For this review, take the finished solid that the model builds, in its own axes (mm). A direction names the side the tool comes from. Coordinates: 2 decimals unless noted, no trailing zeros. Order: outer loops, then holes, each group sorted by start corner. A loop starts at its lowest first (then second) coordinate and runs counter-clockwise, first axis right, second up. Notation, with made-up numbers: (45.5, 85) -> (81.5, 85) arc R20 ccw to (81.5, 112) -> close; hole circle Ø10 at (-16.5, 62). An arc over 180 degrees is marked (long way). Return JSON: item names as keys, results as strings. Group by question number.
Item 1: Take a section at C-C (x = 1262). Write out the cut boundary in (y, z), then the cut area to 3 significant figures.
Item 2: Take a section at A-A (z = -2.5). Write out the cut boundary in (x, y).
Item 3: Take a section at B-B (y = 1). Write out the cut boundary in (x, z).
Item 4: Take a section at D-D (y = -364). Write out the cut boundary in (x, z), then the cut area to 3 significant figures.
Item 5: Insertion check: pin 1 (3 mm diameter, centred on y = -343.5, z = 1.5, fed in from +X); pin 2 (12 mm diameter, centred on y = -415.5, z = -12.5, fed in from -X); pin 3 (15 mm diameter, centred on y = -83.5, z = 6, fed in from -X). Each pin has a flat end and moves straight along its axis. Give the tip position at first contact, or say it passes through.
Item 6: Machinability: for faces 5 (the flat face through (48.573, -44, 1)), 6 (the flat face through (614, 115.552, 1)), which of the approach directions +Z, -Z, +X, -X, +Y, -Y give a long, thin tool a straight path to every point of the face, cutting with its end or side? Answer none if there is none.
Item 7: For line 1 along X through (y, z) = (51.5, 12); line 2 along X through (y, z) = (-128, 1.5); line 3 along X through (y, z) = (-198.5, 5), list the stretches that pass through material, from the lowest coordinate up.
Item 8: Draft analysis for pull direction X (two halves, no side actions). For faces 1 (the flat face through (601, -494.048, 1)), 2 (the flat face through (1166.174, -44, 1)), 3 (the flat face through (23, -190, 1)), 4 (the cylindrical face through (99.346, 111.285, 1.044)), state which applies: +X half, -X half, draft (parallel to the pull), parting line (faces both ways), or undercut.
```python
from build123d import *

# Parameters (mm, degrees)
PAD001_DEPTH = 50.8


with BuildPart() as part:
    # Sketch001 → Pad001 (new body)
    with BuildSketch(Plane.XY):
        with BuildLine():
            Line((-1503.823196, -304.048014), (-589.423152, -304.048014))
            ThreePointArc((-589.423152, -304.048014), (-373.896963, -214.774184), (-284.623087, 0.751986))
            ThreePointArc((-284.623087, 0.751986), (-325.458497, 153.151905), (-437.022924, 264.716435))
            Line((-437.022924, 264.716435), (-437.022924, 0))
            Line((-487.822924, 0), (-437.022924, 0))
            Line((-487.822924, 288.120125), (-487.822924, 0))
            ThreePointArc((-487.822924, 288.120125), (-537.880751, 301.162418), (-589.423152, 305.551986))
            Line((-589.423152, 305.551986), (-1503.823152, 305.551986))
            ThreePointArc((-1503.823152, 305.551986), (-1555.365469, 301.162433), (-1605.423218, 288.120182))
            Line((-1605.423218, 288.120182), (-1605.423218, 0))
            Line((-1656.223218, 0), (-1605.423218, 0))
            Line((-1656.223218, 264.716529), (-1656.223218, 0))
            ThreePointArc((-1656.223218, 264.716529), (-1767.787761, 153.151986), (-1808.623218, 0.751986))
            ThreePointArc((-1808.623218, 0.751986), (-1719.349357, -214.774168), (-1503.823196, -304.048014))
        make_face()
    extrude(amount=PAD001_DEPTH)


with BuildPart() as part_1:
    # Body001 placement: moved
    add(part.part.moved(Location((1653.996692, -189.99962, -23.999952))))


solid = part_1.part
```
Findings below:
{
 "1": {"outline": "(-421.47, -24) -> (42.97, -24) -> (42.97, 26.8) -> (-421.47, 26.8) -> close", "area": "23,600 mm2"},
 "2": {"outline": "(-154.63, -189.25) arc R304.8 ccw to (150.17, -494.05) -> (1064.57, -494.05) arc R304.8 ccw to (1216.97, 74.72) -> (1216.97, -190) -> (1166.17, -190) -> (1166.17, 98.12) arc R304.8 ccw to (1064.57, 115.55) -> (150.17, 115.55) arc R304.8 ccw to (48.57, 98.12) -> (48.57, -190) -> (-2.23, -190) -> (-2.23, 74.72) arc R304.8 ccw to start"},
 "3": {"outline": "(-87.96, -24) -> (-2.23, -24) -> (-2.23, 26.8) -> (-87.96, 26.8) -> close; (48.57, -24) -> (1166.17, -24) -> (1166.17, 26.8) -> (48.57, 26.8) -> close; (1216.97, -24) -> (1302.71, -24) -> (1302.71, 26.8) -> (1216.97, 26.8) -> close"},
 "4": {"outline": "(-99.56, -24) -> (1314.3, -24) -> (1314.3, 26.8) -> (-99.56, 26.8) -> close", "area": "71,800 mm2"},
 "5": {"pin 1": "stops at x = 1328.33", "pin 2": "stops at x = -60.52", "pin 3": "stops at x = -138.36"},
 "6": {"face 5": "+Z, -Z, +Y", "face 6": "+Z, -Z, +X, -X, +Y"},
 "7": {"line 1": "x = -36.76 to -2.23, 48.57 to 1166.17, 1216.97 to 1251.51", "line 2": "x = -148.41 to -2.23, 48.57 to 1166.17, 1216.97 to 1363.16", "line 3": "x = -154.49 to 1369.23"},
 "8": {"face 1": "draft", "face 2": "undercut", "face 3": "undercut", "face 4": "-X half"}
}
